Check sheet for the modelled part. Datum: model origin and axes. Units: mm. Face numbers are marked on the shaded views. Give positions to 0.01 mm unless a question says otherwise; leave off trailing zeros. Write each loop counter-clockwise with the first axis right and the second up, starting at its lowest first coordinate (ties: lowest second). Pieces come first, ordered by that corner, then holes.
from build123d import *

# Parameters (mm, degrees)
SKETCH1_R           = 5.1
BOSS_EXTRUDE1_DEPTH = 4
BOSS_EXTRUDE2_START = -4
BOSS_EXTRUDE2_DEPTH = 4
SKETCH3_R           = 2.5
BOSS_EXTRUDE3_DEPTH = 4
SKETCH4_R           = 1.15
CUT_EXTRUDE1_DEPTH  = 4
FILLET1_R           = 10
FILLET2_R           = 1.5
FILLET3_R           = 5
SKETCH5_W           = 22.86
SKETCH5_H           = 29
BOSS_EXTRUDE4_DEPTH = 4
SKETCH6_W           = 4
SKETCH6_H           = 29
BOSS_EXTRUDE5_DEPTH = 16
FILLET4_R           = 10
FILLET5_R           = 2


with BuildPart() as part:
    # Sketch1 → Boss-Extrude1 (new body)
    with BuildSketch(Plane(origin=(0, 0, 0), x_dir=(1, 0, 0), z_dir=(0, 1, 0))):
        with BuildLine():
            ThreePointArc((-42.589636172, 29.834927363), (-52, 0), (-42.589636172, -29.834927363))
            ThreePointArc((-42.589636172, -29.834927363), (-41.790010768, -41.790010768), (-29.834927363, -42.589636172))
            ThreePointArc((-29.834927363, -42.589636172), (0, -52), (29.834927363, -42.589636172))
            ThreePointArc((29.834927363, -42.589636172), (41.790010768, -41.790010768), (42.589636172, -29.834927363))
            ThreePointArc((42.589636172, -29.834927363), (52, 0), (42.589636172, 29.834927363))
            ThreePointArc((42.589636172, 29.834927363), (41.790010768, 41.790010768), (29.834927363, 42.589636172))
            ThreePointArc((29.834927363, 42.589636172), (0, 52), (-29.834927363, 42.589636172))
            ThreePointArc((-29.834927363, 42.589636172), (-41.790010768, 41.790010768), (-42.589636172, 29.834927363))
        make_face()
        with Locations(Location((-35.355339059, -35.355339059, 0), (0, 0, 270))):
            Circle(SKETCH1_R, mode=Mode.SUBTRACT)
        with Locations(Location((35.355339059, -35.355339059, 0), (0, 0, 270))):
            Circle(SKETCH1_R, mode=Mode.SUBTRACT)
        with BuildLine():
            ThreePointArc((-27.258640426, -39.509068859), (-28.920667351, -28.920667351), (-39.509068859, -27.258640426))
            ThreePointArc((-39.509068859, -27.258640426), (-48, 0), (-39.509068859, 27.258640426))
            ThreePointArc((-39.509068859, 27.258640426), (-28.920667351, 28.920667351), (-27.258640426, 39.509068859))
            ThreePointArc((-27.258640426, 39.509068859), (0, 48), (27.258640426, 39.509068859))
            ThreePointArc((27.258640426, 39.509068859), (28.920667351, 28.920667351), (39.509068859, 27.258640426))
            ThreePointArc((39.509068859, 27.258640426), (48, 0), (39.509068859, -27.258640426))
            ThreePointArc((39.509068859, -27.258640426), (28.920667351, -28.920667351), (27.258640426, -39.509068859))
            ThreePointArc((27.258640426, -39.509068859), (0, -48), (-27.258640426, -39.509068859))
        make_face(mode=Mode.SUBTRACT)
        with Locations(Location((-35.355339059, 35.355339059, 0), (0, 0, 270))):
            Circle(SKETCH1_R, mode=Mode.SUBTRACT)
        with Locations(Location((35.355339059, 35.355339059, 0), (0, 0, 270))):
            Circle(SKETCH1_R, mode=Mode.SUBTRACT)
    extrude(amount=BOSS_EXTRUDE1_DEPTH)

    # Sketch2 → Boss-Extrude2 (add)
    with BuildSketch(Plane(origin=(0, 4, 0), x_dir=(1, 0, 0), z_dir=(0, 1, 0)).offset(BOSS_EXTRUDE2_START)):
        with BuildLine():
            ThreePointArc((-26.255339059, 35.355339059), (-26.311135203, 34.349169788), (-26.477839411, 33.355339059))
            Line((-26.477839411, 33.355339059), (26.477839411, 33.355339059))
            ThreePointArc((26.477839411, 33.355339059), (26.255339059, 35.355339059), (26.477839411, 37.355339059))
            Line((26.477839411, 37.355339059), (-26.477839411, 37.355339059))
            ThreePointArc((-26.477839411, 37.355339059), (-26.311135203, 36.36150833), (-26.255339059, 35.355339059))
        make_face()
        with BuildLine():
            Line((-33.355339059, -26.477839411), (-33.355339059, 26.477839411))
            ThreePointArc((-33.355339059, 26.477839411), (-35.355339059, 26.255339059), (-37.355339059, 26.477839411))
            Line((-37.355339059, 26.477839411), (-37.355339059, -26.477839411))
            ThreePointArc((-37.355339059, -26.477839411), (-35.355339059, -26.255339059), (-33.355339059, -26.477839411))
        make_face()
        with BuildLine():
            ThreePointArc((37.355339059, 26.477839411), (35.355339059, 26.255339059), (33.355339059, 26.477839411))
            Line((33.355339059, 26.477839411), (33.355339059, -26.477839411))
            ThreePointArc((33.355339059, -26.477839411), (35.355339059, -26.255339059), (37.355339059, -26.477839411))
            Line((37.355339059, -26.477839411), (37.355339059, 26.477839411))
        make_face()
        with BuildLine():
            Line((26.477839411, -33.355339059), (-26.477839411, -33.355339059))
            ThreePointArc((-26.477839411, -33.355339059), (-26.311135203, -34.349169788), (-26.255339059, -35.355339059))
            ThreePointArc((-26.255339059, -35.355339059), (-26.311135203, -36.36150833), (-26.477839411, -37.355339059))
            Line((-26.477839411, -37.355339059), (26.477839411, -37.355339059))
            ThreePointArc((26.477839411, -37.355339059), (26.255339059, -35.355339059), (26.477839411, -33.355339059))
        make_face()
    extrude(amount=BOSS_EXTRUDE2_DEPTH)

    # Sketch3 → Boss-Extrude3 (add)
    with BuildSketch(Plane(origin=(0, 4, 0), x_dir=(1, 0, 0), z_dir=(0, 1, 0))):
        with Locations((-20, 35.355339059)):
            Circle(SKETCH3_R)
        with Locations((20, 35.355339059)):
            Circle(SKETCH3_R)
        with Locations((35.355339059, 20)):
            Circle(SKETCH3_R)
        with Locations((35.355339059, -20)):
            Circle(SKETCH3_R)
        with Locations((-35.355339059, -20)):
            Circle(SKETCH3_R)
        with Locations((-35.355339059, 20)):
            Circle(SKETCH3_R)
        with Locations((-20, -35.355339059)):
            Circle(SKETCH3_R)
        with Locations((20, -35.355339059)):
            Circle(SKETCH3_R)
    extrude(amount=-BOSS_EXTRUDE3_DEPTH)

    # Sketch4 → Cut-Extrude1 (cut)
    with BuildSketch(Plane(origin=(0, 4, 0), x_dir=(1, 0, 0), z_dir=(0, 1, 0))):
        with Locations(Location((-20, 35.355339059, 0), (0, 0, 270))):
            Circle(SKETCH4_R)
        with Locations(Location((20, 35.355339059, 0), (0, 0, 270))):
            Circle(SKETCH4_R)
        with Locations(Location((-35.355339059, 20, 0), (0, 0, 270))):
            Circle(SKETCH4_R)
        with Locations(Location((-35.355339059, -20, 0), (0, 0, 270))):
            Circle(SKETCH4_R)
        with Locations(Location((-20, -35.355339059, 0), (0, 0, 270))):
            Circle(SKETCH4_R)
        with Locations(Location((20, -35.355339059, 0), (0, 0, 270))):
            Circle(SKETCH4_R)
        with Locations(Location((35.355339059, -20, 0), (0, 0, 270))):
            Circle(SKETCH4_R)
        with Locations(Location((35.355339059, 20, 0), (0, 0, 270))):
            Circle(SKETCH4_R)
    extrude(amount=-CUT_EXTRUDE1_DEPTH, mode=Mode.SUBTRACT)

    # Fillet1
    fillet1_edges = [part.edges().sort_by_distance(p)[0] for p in [
        (-42.589636172, 2, 29.834927363),
        (-42.589636172, 2, -29.834927363),
        (-29.834927363, 2, -42.589636172),
        (29.834927363, 2, -42.589636172),
        (42.589636172, 2, -29.834927363),
        (42.589636172, 2, 29.834927363),
        (29.834927363, 2, 42.589636172),
        (-29.834927363, 2, 42.589636172),
    ]]
    fillet(fillet1_edges, radius=FILLET1_R)

    # Fillet2
    fillet2_edges = [part.edges().sort_by_distance(p)[0] for p in [
        (37.355339059, 2, -26.477839411),
        (37.355339059, 2, 26.477839411),
        (-26.477839411, 2, 37.355339059),
        (26.477839411, 2, 37.355339059),
        (27.258640426, 2, 39.509068859),
        (39.509068859, 2, 27.258640426),
        (39.509068859, 2, -27.258640426),
        (27.258640426, 2, -39.509068859),
        (-27.258640426, 2, -39.509068859),
        (-39.509068859, 2, -27.258640426),
        (-39.509068859, 2, 27.258640426),
        (-27.258640426, 2, 39.509068859),
        (-26.477839411, 2, -37.355339059),
        (26.477839411, 2, -37.355339059),
        (-37.355339059, 2, -26.477839411),
        (-37.355339059, 2, 26.477839411),
    ]]
    fillet(fillet2_edges, radius=FILLET2_R)

    # Fillet3
    fillet3_edges = [part.edges().sort_by_distance(p)[0] for p in [
        (33.355339059, 2, -26.477839411),
        (33.355339059, 2, 26.477839411),
        (-26.477839411, 2, 33.355339059),
        (26.477839411, 2, 33.355339059),
        (-26.477839411, 2, -33.355339059),
        (26.477839411, 2, -33.355339059),
        (-33.355339059, 2, -26.477839411),
        (-33.355339059, 2, 26.477839411),
    ]]
    fillet(fillet3_edges, radius=FILLET3_R)

    # Sketch5 → Boss-Extrude4 (add)
    with BuildSketch(Plane(origin=(0, 4, 0), x_dir=(1, 0, 0), z_dir=(0, 1, 0))):
        with Locations((21.925339059, 0)):
            Rectangle(SKETCH5_W, SKETCH5_H)
    extrude(amount=-BOSS_EXTRUDE4_DEPTH)

    # Sketch6 → Boss-Extrude5 (add)
    with BuildSketch(Plane.XZ):
        with Locations((12.495339059, 0)):
            Rectangle(SKETCH6_W, SKETCH6_H)
    extrude(amount=-BOSS_EXTRUDE5_DEPTH)

    # Fillet4
    # the kernel refuses this fillet: 10 mm, written as the material it takes off along each edge
    with BuildSketch(Plane(origin=(14.495339059, 4, -14.5), x_dir=(0, 0, 1), z_dir=(0, 1, 0))) as fillet4_piece_1:
        with BuildLine():
            CenterArc((8, -10), FILLET4_R, 90, 53.130102354)
            Line((0, -4), (0, 0))
            Line((0, 0), (8, 0))
        make_face()
    extrude(amount=32, mode=Mode.SUBTRACT)
    with BuildSketch(Plane(origin=(14.495339059, 4, 14.5), x_dir=(0, 0, -1), z_dir=(0, 1, 0))) as fillet4_piece_2:
        with BuildLine():
            CenterArc((8, 10), FILLET4_R, 216.869897646, 53.130102354)
            Line((0, 4), (0, 0))
            Line((0, 0), (8, 0))
        make_face()
    extrude(amount=32, mode=Mode.SUBTRACT)

    # Fillet5
    fillet5_edges = [part.edges().sort_by_distance(p)[0] for p in [
        (33.355339059, 0, 16.5),
        (33.355339059, 2, -14.5),
        (21.925339059, 0, 14.5),
        (33.355339059, 2, 14.5),
        (21.925339059, 0, -14.5),
        (33.355339059, 0, -16.5),
    ]]
    fillet(fillet5_edges, radius=FILLET5_R)


solid = part.part
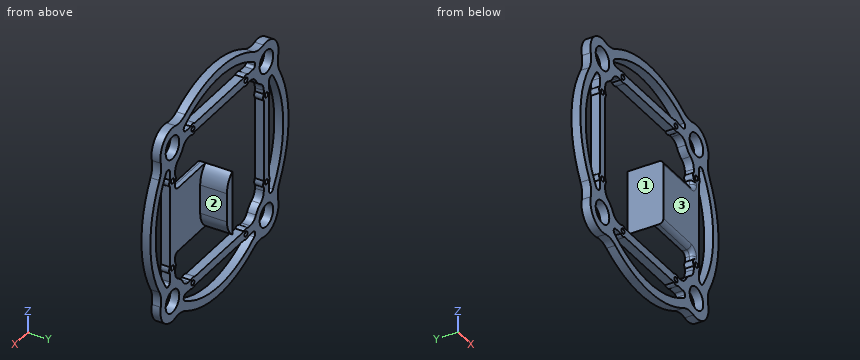
1) Scan lines: L1, parallel to Z at x = 8, y = 2; L2, parallel to Y at x = 30.5, z = 38.5; L3, parallel to Z at x = 28, y = 2.5. Record each from-to range of solid material in increasing order.
2) Sectioned sample at B-B on y = 11.5. Record the boundary of the cut face in (x, z).
3) Gauge pin test, flat ends, axial feed: pin 1 (6 mm diameter, centred on y = 6, z = -28, fed in from -X); pin 2 (1 mm diameter, centred on x = 16, y = 6, fed in from -Z); pin 3 (4.5 mm diameter, centred on y = 2, z = -7, fed in from -X); pin 4 (0.6 mm diameter, centred on y = 3, z = -17, fed in from -X). Record the tip position at first contact, or that the pin passes through.
4) Sectioned sample at A-A on x = -7. Record the boundary of the cut face in (y, z).
5) Draft check along X on the marked faces 1, 2 and 3. Enter one of: +X half, -X half, draft (parallel to the pull), parting line (faces both ways), or undercut.
Answers below:
1. L1: z = -51.38 to -47.33, -37.36 to -33.36, 33.36 to 37.36, 47.33 to 51.38
1. L2: y = 0 to 4
1. L3: z = -44.24 to -30, -14.5 to 14.5, 30 to 44.24
2. outline: (10.5, -14.5) arc R10 ccw to (14.5, -6.5) - (14.5, 6.5) arc R10 ccw to (10.5, 14.5) - close
3. pin 1: stops at x = -45.17
3. pin 2: passes through
3. pin 3: stops at x = -51.78
3. pin 4: stops at x = -49.25
4. outline: (0, -51.53) - (4, -51.53) - (4, -47.49) - (0, -47.49) - close; (0, -37.36) - (4, -37.36) - (4, -33.36) - (0, -33.36) - close; (0, 33.36) - (4, 33.36) - (4, 37.36) - (0, 37.36) - close; (0, 47.49) - (4, 47.49) - (4, 51.53) - (0, 51.53) - close
5. face 1: undercut
5. face 2: +X half
5. face 3: draft
